```python
from build123d import *

# Parameters (mm, degrees)
F0_R     = 2.5
F1_DEPTH = 15
F2_R     = 6.5
F3_DEPTH = 3
F4_SIZE  = 2


with BuildPart() as f1:
    # F0 (on Top) → F1 (new body)
    with BuildSketch(Plane.XY):
        Polygon((15, 0.599955), (15, 2.061703), (14.605625, 3.469245), (10.659539, 2.727035), (10.524641, 3.208494), (14.281893, 4.624658), (13.887519, 6.032201), (13.128018, 7.281146), (9.528509, 5.501819), (9.268717, 5.929028), (12.504564, 8.306372), (11.745064, 9.555318), (10.676766, 10.553039), (7.690794, 7.868557), (7.325376, 8.209834), (9.799829, 11.37204), (8.731531, 12.369761), (7.433666, 13.04226), (5.282687, 9.651721), (4.838744, 9.881754), (6.368285, 13.594296), (5.07042, 14.266796), (3.639246, 14.564197), (2.482787, 10.719061), (1.993245, 10.820789), (2.464434, 14.808326), (1.03326, 15.105727), (-0.42508, 15.005974), (-0.501249, 10.991417), (-1.000084, 10.957296), (-1.622192, 14.924089), (-3.080532, 14.824336), (-4.45788, 14.334826), (-3.448111, 10.44859), (-3.919241, 10.28115), (-5.588508, 13.933001), (-6.965856, 13.443492), (-8.16006, 12.60053), (-6.139241, 9.130839), (-6.547726, 8.842499), (-9.14035, 11.908566), (-10.334554, 11.065605), (-11.257045, 9.931711), (-8.375052, 7.135895), (-8.690596, 6.74804), (-12.014294, 9.000928), (-12.936785, 7.867033), (-13.519147, 6.526302), (-9.989724, 4.611715), (-10.188925, 4.153109), (-13.997192, 5.425731), (-14.579554, 4.084999), (-14.778595, 2.636866), (-10.863504, 1.745505), (-10.931587, 1.250162), (-14.941983, 1.448133), (-15.141024, 0), (-14.941983, -1.448133), (-10.931587, -1.250162), (-10.863504, -1.745505), (-14.778595, -2.636866), (-14.579554, -4.084999), (-13.997192, -5.425731), (-10.188925, -4.153109), (-9.989724, -4.611715), (-13.519147, -6.526302), (-12.936785, -7.867033), (-12.014294, -9.000928), (-8.690596, -6.74804), (-8.375052, -7.135895), (-11.257045, -9.931711), (-10.334554, -11.065605), (-9.14035, -11.908566), (-6.547726, -8.842499), (-6.139241, -9.130839), (-8.16006, -12.60053), (-6.965856, -13.443492), (-5.588508, -13.933001), (-3.919241, -10.28115), (-3.448111, -10.44859), (-4.45788, -14.334826), (-3.080532, -14.824336), (-1.622192, -14.924089), (-1.000084, -10.957296), (-0.501249, -10.991417), (-0.42508, -15.005974), (1.03326, -15.105727), (2.464434, -14.808326), (1.993245, -10.820789), (2.482787, -10.719061), (3.639246, -14.564197), (5.07042, -14.266796), (6.368285, -13.594296), (4.838744, -9.881754), (5.282687, -9.651721), (7.433666, -13.04226), (8.731531, -12.369761), (9.799829, -11.37204), (7.325376, -8.209834), (7.690794, -7.868557), (10.676766, -10.553039), (11.745064, -9.555318), (12.504564, -8.306372), (9.268717, -5.929028), (9.528509, -5.501819), (13.128018, -7.281146), (13.887519, -6.032201), (14.281893, -4.624658), (10.524641, -3.208494), (10.659539, -2.727035), (14.605625, -3.469245), (15, -2.061703), (15, -0.599955), (11, -0.25), (11, 0.25), align=None)
        Circle(F0_R, mode=Mode.SUBTRACT)
    extrude(amount=F1_DEPTH)

    # F2 (on face) → F3 (cut)
    with BuildSketch(Plane(origin=(0, 0, 0), x_dir=(1, 0, 0), z_dir=(0, 0, -1))):
        Circle(F2_R)
    extrude(amount=-F3_DEPTH, mode=Mode.SUBTRACT)

    # F4
    f4_edges = [f1.edges().sort_by_distance(p)[0] for p in [
        (-2.5, 0, 15),
    ]]
    chamfer(f4_edges, length=F4_SIZE)


solid = f1.part
```
Source: CAD feature listing. Evaluate the final solid. Frame: model axes, mm. A direction names the side the tool comes from. Round coordinates to 2 decimals unless told otherwise and drop trailing zeros. Write each loop counter-clockwise with the first axis right and the second up, starting at its lowest first coordinate (ties: lowest second). Pieces come first, ordered by that corner, then holes. Notation, with made-up numbers: M 65.5,74.25 L 84.5,74.25 A11 ccw 84.5,92.25 Z; hole C 43.5,70 d5. An arc over 180 degrees is marked long. Answer as a JSON object with one key per item and string values. Group by question number.
(1) Ray query, line 1 (X direction, y = 0, z = 1.7); line 2 (X direction, y = 0, z = 6.25); line 3 (X direction, y = -12, z = 2.5). Return the intervals inside material, ascending. Write a range as [from, to].
(2) First-contact query: pin 1 (6 mm diameter, centred on x = -4, z = 3, fed in from -Y); pin 2 (8 mm diameter, centred on x = 0, y = 0, fed in from +Z); pin 3 (2 mm diameter, centred on y = 4, z = 6, fed in from -X); pin 4 (6 mm diameter, centred on x = 6, y = 1, fed in from -Z). Flat tips, straight axial feed; report the tip coordinate or a pass-through.
(3) Reachability of faces 5 (the flat face through (3.07, 12.67, 7.4)), 6 (the flat face through (-1.315, -12.968, 7.395)), 7 (the flat face through (11.303, -6.379, 7.395)), 8 (the flat face through (-14.678, 3.371, 7.395)) from +Z, -Z, +X, -X, +Y, -Y: full face, straight path, thin tool, end or side. Return the list, or none.
(4) Section query A-A on x = 0. Output: boundary loops of the cut face in (y, z), then the cut area to 3 significant figures.
(5) Mould query, pull axis Y, two halves, no side actions, for faces 1 (the flat face through (13.5, -6.67, 7.4)), 2 (the flat face through (12.6, -3.09, 7.4)), 3 (the flat face through (6.34, -11.32, 7.4)), 4 (the flat face through (4.365, 14.413, 7.395)). Classes: +Y half, -Y half, draft (parallel to the pull), parting line (faces both ways), or undercut.
Computed values:
{
 "1": {"line 1": "[-15.14, -6.5], [6.5, 11]", "line 2": "[-15.14, -2.5], [2.5, 11]", "line 3": "[-7.81, -4.7], [-3.85, -1.16], [-0.48, 2.13], [2.87, 5.71], [6.77, 9.13]"},
 "2": {"pin 1": "y = -14.92", "pin 2": "z = 14.5", "pin 3": "x = -14.73", "pin 4": "z = 0"},
 "3": {"face 5": "+Z, -Z, +Y", "face 6": "+Z, -Z, -Y", "face 7": "+Z, -Z", "face 8": "+Z, -Z, -X, +Y"},
 "4": {"outline": "M -15.04,0 L -6.5,0 L -6.5,3 L -2.5,3 L -2.5,13 L -4.5,15 L -15.04,15 Z; M 2.5,3 L 6.5,3 L 6.5,0 L 15.04,0 L 15.04,15 L 4.5,15 L 2.5,13 Z", "area": "348 mm^2"},
 "5": {"face 1": "-Y half", "face 2": "undercut", "face 3": "undercut", "face 4": "+Y half"}
}
